The listing builds one solid part. Answer for the finished solid, in the listing's coordinates (mm). Face numbers are marked on the shaded views. A direction names the side the tool comes from. Coordinates: 2 decimals unless noted, no trailing zeros. Write each loop counter-clockwise with the first axis right and the second up, starting at its lowest first coordinate (ties: lowest second). Pieces come first, ordered by that corner, then holes.
(1) The part is cut by section A-A on y = -12.5. Determine the outline of the cut face in (x, z), plus the area to 3 significant figures.
(2) Which of the six approach directions +Z, -Z, +X, -X, +Y, -Y give full straight-line access (tool end or side, diameter ignored) to the marked faces 1, 2 and 3?
(3) The part is cut by section B-B on x = 0. Determine the outline of the cut face in (y, z).
(4) For a pull along X with two mould halves and no side action, classify the marked faces 4, 5 and 6 as +X half, -X half, draft (parallel to the pull), parting line (faces both ways), or undercut.
(5) Straight lines are drawn through the part: line 1 (Y direction, x = 0, z = 2.15); line 2 (Y direction, x = 0, z = -3); line 3 (X direction, y = -18.5, z = 2.75). For each, find the intervals that lie inside material, in ascending order.
(6) Given P1, Ø1, axis at y = 30, z = -1, coming from the -X side; P2, Ø20, axis at x = 0, y = 0, coming from the -Z side; P3, Ø4, axis at x = 28, z = 2, coming from the -Y side; P4, Ø1, axis at x = 16, z = 0.5, coming from the -Y side, each flat-ended and moving along its own axis, determine where each tip first touches the part or whether it passes through.
from build123d import *

# Parameters (mm, degrees)
F0_R     = 11
F1_DEPTH = 3.5
F2_R     = 1
F3_R     = 1


# Not quite as in the source:
# - a feature names something its author has since deleted; it is built from what else it names


with BuildPart() as f1:
    # F0 (on Top) → F1 (new body, symmetric)
    with BuildSketch(Plane.XY):
        with BuildLine():
            ThreePointArc((-28.6506350946, -0.375644347), (-33.7749907476, -19.5), (-14.6506350946, -24.624355653))
            Line((-14.6506350946, -24.624355653), (-2.5, -17.6091832103))
            ThreePointArc((-2.5, -17.6091832103), (0, -16.9393102292), (2.5, -17.6091832103))
            Line((2.5, -17.6091832103), (14.6506350946, -24.624355653))
            ThreePointArc((14.6506350946, -24.624355653), (33.7749907476, -19.5), (28.6506350946, -0.375644347))
            Line((28.6506350946, -0.375644347), (16.5, 6.6395280957))
            ThreePointArc((16.5, 6.6395280957), (14.6698729811, 8.4696551146), (14, 10.9696551146))
            Line((14, 10.9696551146), (14, 25))
            ThreePointArc((14, 25), (0, 39), (-14, 25))
            Line((-14, 25), (-14, 10.9696551146))
            ThreePointArc((-14, 10.9696551146), (-14.6698729811, 8.4696551146), (-16.5, 6.6395280957))
            Line((-16.5, 6.6395280957), (-28.6506350946, -0.375644347))
        make_face()
        with Locations((-21.6506350946, -12.5)):
            Circle(F0_R, mode=Mode.SUBTRACT)
        with Locations((21.6506350946, -12.5)):
            Circle(F0_R, mode=Mode.SUBTRACT)
        Circle(F0_R, mode=Mode.SUBTRACT)
        with Locations((0, 25)):
            Circle(F0_R, mode=Mode.SUBTRACT)
    extrude(amount=F1_DEPTH, both=True)

    # F2
    f2_edges = [f1.edges().sort_by_distance(p)[0] for p in [
        (-8.575318, -21.116769, 3.5),
        (-33.774991, -19.5, 3.5),
        (-22.575318, 3.131942, 3.5),
    ]]
    fillet(f2_edges, radius=F2_R)

    # F3
    f3_edges = [f1.edges().sort_by_distance(p)[0] for p in [
        (-8.575318, -21.116769, -3.5),
        (-33.774991, -19.5, -3.5),
        (-22.575318, 3.131942, -3.5),
        (-11, 25, -3.5),
    ]]
    fillet(f3_edges, radius=F3_R)


solid = f1.part
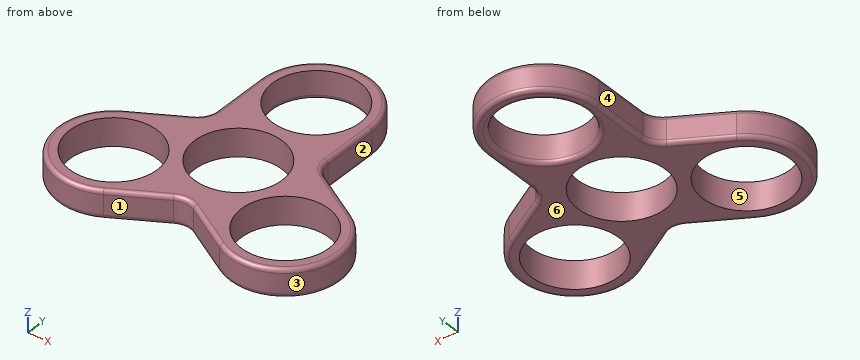
Model answer:
1. outline: (-35.65, -2.5) arc R1 ccw to (-34.65, -3.5) - (-32.65, -3.5) - (-32.65, 3.5) - (-34.65, 3.5) arc R1 ccw to (-35.65, 2.5) - close; (-10.65, -3.5) - (10.65, -3.5) - (10.65, 3.5) - (-10.65, 3.5) - close; (32.65, -3.5) - (34.65, -3.5) arc R1 ccw to (35.65, -2.5) - (35.65, 2.5) arc R1 ccw to (34.65, 3.5) - (32.65, 3.5) - close
1. area: 190 mm2
2. face 1: +Z, -Z, -Y
2. face 2: +Z, -Z, +X, +Y
2. face 3: +Z, -Z
3. outline: (-16.94, -2.5) arc R1 ccw to (-15.94, -3.5) - (-11, -3.5) - (-11, 3.5) - (-15.94, 3.5) arc R1 ccw to (-16.94, 2.5) - close; (11, -3.5) - (13, -3.5) arc R1 ccw to (14, -2.5) - (14, 3.5) - (11, 3.5) - close; (36, -2.5) arc R1 ccw to (37, -3.5) - (38, -3.5) arc R1 ccw to (39, -2.5) - (39, 2.5) arc R1 ccw to (38, 3.5) - (36, 3.5) - close
4. face 4: -X half
4. face 5: undercut
4. face 6: draft
5. line 1: y = -16.94 to -11, 11 to 14, 36 to 39
5. line 2: y = -16.81 to -11, 11 to 13.87, 36.13 to 38.87
5. line 3: x = -34.26 to -30.87, -12.43 to -4.11, 4.11 to 12.43, 30.87 to 34.26
6. P1: stops at x = -13.26
6. P2: passes through
6. P3: stops at y = -25.81
6. P4: stops at y = -25.52
